from build123d import *

# Parameters (mm, degrees)
SKETCH_1_W      = 64
SKETCH_1_H      = 7.5
SKETCH_1_R      = 7.5
SKETCH_1_R_2    = 5
EXTRUDE_1_DEPTH = 8
FILLET_1_R      = 3


with BuildPart() as part:
    # 草图1 → 凸台-拉伸1 (new body)
    # profile 1 of 3: a face of its own
    with BuildSketch(Plane(origin=(0, 0, 0), x_dir=(1, 0, 0), z_dir=(0, 1, 0))):
        with BuildLine():
            Line((165, 7.5), (0, 7.5))
            ThreePointArc((0, 7.5), (5.303300859, 5.303300859), (7.5, 0))
            ThreePointArc((7.5, 0), (5.303300859, -5.303300859), (0, -7.5))
            Line((0, -7.5), (165, -7.5))
            ThreePointArc((165, -7.5), (157.5, 0), (165, 7.5))
        make_face()
        with Locations((46.5, 0)):
            Rectangle(SKETCH_1_W, SKETCH_1_H, mode=Mode.SUBTRACT)
        with Locations((118.5, 0)):
            Rectangle(SKETCH_1_W, SKETCH_1_H, mode=Mode.SUBTRACT)
    # profile 2 of 3: a face of its own
    with BuildSketch(Plane(origin=(0, 0, 0), x_dir=(1, 0, 0), z_dir=(0, 1, 0))):
        Circle(SKETCH_1_R)
        with Locations(Location((0, 0, 0), (0, 0, 270))):
            Circle(SKETCH_1_R_2, mode=Mode.SUBTRACT)
    # profile 3 of 3: a face of its own
    with BuildSketch(Plane(origin=(0, 0, 0), x_dir=(1, 0, 0), z_dir=(0, 1, 0))):
        with Locations((165, 0)):
            Circle(SKETCH_1_R)
        with Locations(Location((165, 0, 0), (0, 0, 270))):
            Circle(SKETCH_1_R_2, mode=Mode.SUBTRACT)
    extrude(amount=EXTRUDE_1_DEPTH)

    # 圆角1
    fillet_1_edges = [part.edges().sort_by_distance(p)[0] for p in [
        (86.5, 4, -3.75),
        (86.5, 4, 3.75),
        (150.5, 4, 3.75),
        (150.5, 4, -3.75),
        (14.5, 4, -3.75),
        (14.5, 4, 3.75),
        (78.5, 4, 3.75),
        (78.5, 4, -3.75),
    ]]
    fillet(fillet_1_edges, radius=FILLET_1_R)


solid = part.part
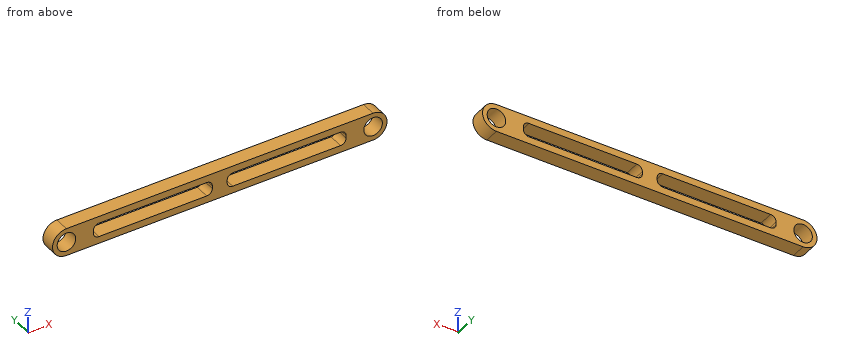
Could you check a few things on this model? Use its own coordinates, in mm. Give positions to 0.01 mm unless a question says otherwise; leave off trailing zeros. Order: outer loops, then holes, each group sorted by start corner. A loop starts at its lowest first (then second) coordinate and runs counter-clockwise, first axis right, second up. Notation, with made-up numbers: (-22, -21) - (10, -21) arc R31 cw to (10, 5) - close; hole circle Ø5 at (-5.75, -7). An arc over 180 degrees is marked (long way). Return JSON: item names as keys, results as strings. Group by question number.
Q1. Please list where these lines run through material, in increasing order: line 1 along X through (y, z) = (3.75, 0); line 2 along Z through (x, y) = (71, 2); line 3 along X through (y, z) = (3.25, 1.5). Write a range as [from, to].
Q2. Suppose I cut it at B-B, the plane y = 1.5. Please give me the cut outline in (x, z), and give its area (3 significant figures).
Q3. Suppose I cut it at A-A, the plane x = 67. Please give me the cut outline in (y, z).
Q4. Will these pins go through, and if not, where does the flat tip stop? pin 1 Ø8 at (x, z) = (0, 0) entering from +Y; pin 2 Ø1 at (y, z) = (4.5, -3) entering from +X.
Resolved:
{
 "1": {"line 1": "x = [-7.5, -5], [5, 14.5], [78.5, 86.5], [150.5, 160], [170, 172.5]", "line 2": "z = [-7.5, -3.75], [3.75, 7.5]", "line 3": "x = [-7.35, -4.77], [4.77, 14.6], [78.4, 86.6], [150.4, 160.23], [169.77, 172.35]"},
 "2": {"outline": "(0, -7.5) - (165, -7.5) arc R7.5 ccw to (165, 7.5) - (0, 7.5) arc R7.5 ccw to start; hole circle Ø10 at (0, 0); hole (14.5, -0.75) arc R3 ccw to (17.5, -3.75) - (75.5, -3.75) arc R3 ccw to (78.5, -0.75) - (78.5, 0.75) arc R3 ccw to (75.5, 3.75) - (17.5, 3.75) arc R3 ccw to (14.5, 0.75) - close; hole (86.5, -0.75) arc R3 ccw to (89.5, -3.75) - (147.5, -3.75) arc R3 ccw to (150.5, -0.75) - (150.5, 0.75) arc R3 ccw to (147.5, 3.75) - (89.5, 3.75) arc R3 ccw to (86.5, 0.75) - close; hole circle Ø10 at (165, 0)", "area": "1,550 mm2"},
 "3": {"outline": "(0, -7.5) - (8, -7.5) - (8, -3.75) - (0, -3.75) - close; (0, 3.75) - (8, 3.75) - (8, 7.5) - (0, 7.5) - close"},
 "4": {"pin 1": "passes through", "pin 2": "stops at x = 172.07"}
}
